Here's how the part is built. I have some questions about the finished solid (model axes, mm). A direction names the side the tool comes from. Give positions to 0.01 mm unless a question says otherwise; leave off trailing zeros. Write each loop counter-clockwise with the first axis right and the second up, starting at its lowest first coordinate (ties: lowest second). Pieces come first, ordered by that corner, then holes. Notation, with made-up numbers: (-22.5, -4) - (-5.5, -4) arc R15 cw to (-5.5, 7) - close; hole circle Ø9 at (8, 31.5). An arc over 180 degrees is marked (long way). Use a Markdown table: item, result.
```python
from build123d import *

# Parameters (mm, degrees)
BOX001_W               = 10
BOX001_H               = 20
BOX001_DEPTH           = 10
BOX001_PLACEMENT_ANGLE = 315
BOX_W                  = 10
BOX_H                  = 20
BOX_DEPTH              = 10


with BuildPart() as cubo001:
    # Box001 → Box001 (new body)
    with BuildSketch(Plane.XY):
        with Locations((5, 10)):
            Rectangle(BOX001_W, BOX001_H)
    extrude(amount=BOX001_DEPTH)


with BuildPart() as cubo001_1:
    # Box001 placement: moved
    add(cubo001.part.moved(Location((0, -10, 3))).rotate(Axis((0, -10, 3), (0, 1, 0)), BOX001_PLACEMENT_ANGLE))


with BuildPart() as fusion:
    # Box → Box (new body)
    with BuildSketch(Plane(origin=(-5, -10, 0), x_dir=(1, 0, 0), z_dir=(0, 0, 1))):
        with Locations((5, 10)):
            Rectangle(BOX_W, BOX_H)
    extrude(amount=BOX_DEPTH)

    # Fusion: union Cubo001
    add(cubo001_1.part)


solid = fusion.part
```
Item 1: If we section it at C-C, the plane x = -3.25: Write out the boundary of the cut face in (y, z), plus the area to 3 significant figures.
Values:
| item | result |
|---|---|
| outline | (-10, 0) - (10, 0) - (10, 13.89) - (-10, 13.89) - close |
| area | 278 mm2 |
Item 2: For faces 1 (the flat face through (0, 0, 0)), 2 (the flat face through (-5, 0, 4)), 3 (the flat face through (5, 0, 4)), which set-ups out of +Z, -Z, +X, -X, +Y, -Y let a thin tool reach every point of the face, with its end or its side?
Values:
| item | result |
|---|---|
| face 1 | -Z, +X, -X, +Y, -Y |
| face 2 | -Z, -X, +Y, -Y |
| face 3 | -Z, +X, +Y, -Y |
Item 3: If we section it at A-A, the plane y = 8.5: Write out the boundary of the cut face in (x, z), plus the area to 3 significant figures.
Values:
| item | result |
|---|---|
| outline | (-7.07, 10.07) - (-5, 8) - (-5, 0) - (5, 0) - (5, 8) - (7.07, 10.07) - (0, 17.14) - close |
| area | 155 mm2 |
Item 4: I need wall thicknesses on line 1 along X through (y, z) = (4.25, 1.75); line 2 along X through (y, z) = (0, 15.25); line 3 along Z through (x, y) = (5.75, -5). Which ranges of each line are inside material? Lowest first, please. Write a range as [from, to].
Values:
| item | result |
|---|---|
| line 1 | x = [-5, 5] |
| line 2 | x = [-1.89, 1.89] |
| line 3 | z = [8.75, 11.39] |
Item 5: If we section it at B-B, the plane z = 5.5: Write out the boundary of the cut face in (x, y).
Values:
| item | result |
|---|---|
| outline | (-5, -10) - (5, -10) - (5, 10) - (-5, 10) - close |
Item 6: Will these pins go through, and if not, where does the flat tip stop? pin 1 Ø10 at (y, z) = (-0.5, 4) entering from -X; pin 2 Ø6 at (x, y) = (5, 6.5) entering from -Z; pin 3 Ø1 at (x, y) = (4, -3) entering from +Z; pin 4 Ø9 at (y, z) = (-0.5, 4) entering from +X.
Values:
| item | result |
|---|---|
| pin 1 | stops at x = -6 |
| pin 2 | stops at z = 0 |
| pin 3 | stops at z = 13.64 |
| pin 4 | stops at x = 5.5 |
